```python
from build123d import *

# Parameters (mm, degrees)
F0_R     = 20
F1_DEPTH = 2
F2_R     = 5
F2_R_2   = 1.1
F3_DEPTH = 1.5


with BuildPart() as f1:
    # F0 (on Top) → F1 (new body)
    with BuildSketch(Plane.XY):
        Circle(F0_R)
        Polygon((-10.984643, -14.268413), (-5.694576, -6.98726), (-5.290067, -7.281153), (-4.885559, -7.575046), (-10.175626, -14.856199), (-10.580135, -14.562306), align=None, mode=Mode.SUBTRACT)
        Polygon((-6.037834, -16.964509), (-3.256681, -8.405), (-2.781153, -8.559509), (-2.305625, -8.714017), (-5.086778, -17.273526), (-5.562306, -17.119017), align=None, mode=Mode.SUBTRACT)
        Polygon((-14.856199, -10.175626), (-7.575046, -4.885559), (-7.281153, -5.290067), (-6.98726, -5.694576), (-14.268413, -10.984643), (-14.562306, -10.580135), align=None, mode=Mode.SUBTRACT)
        Polygon((-17.273526, -5.086778), (-8.714017, -2.305625), (-8.559509, -2.781153), (-8.405, -3.256681), (-16.964509, -6.037834), (-17.119017, -5.562306), align=None, mode=Mode.SUBTRACT)
        Polygon((-0.5, -9), (0, -9), (0.5, -9), (0.5, -18), (0, -18), (-0.5, -18), align=None, mode=Mode.SUBTRACT)
        Polygon((5.086778, -17.273526), (2.305625, -8.714017), (2.781153, -8.559509), (3.256681, -8.405), (6.037834, -16.964509), (5.562306, -17.119017), align=None, mode=Mode.SUBTRACT)
        Polygon((10.175626, -14.856199), (4.885559, -7.575046), (5.290067, -7.281153), (5.694576, -6.98726), (10.984643, -14.268413), (10.580135, -14.562306), align=None, mode=Mode.SUBTRACT)
        Polygon((14.268413, -10.984643), (6.98726, -5.694576), (7.281153, -5.290067), (7.575046, -4.885559), (14.856199, -10.175626), (14.562306, -10.580135), align=None, mode=Mode.SUBTRACT)
        Polygon((16.964509, -6.037834), (8.405, -3.256681), (8.559509, -2.781153), (8.714017, -2.305625), (17.273526, -5.086778), (17.119017, -5.562306), align=None, mode=Mode.SUBTRACT)
        Polygon((-18, 0.5), (-9, 0.5), (-9, 0), (-9, -0.5), (-18, -0.5), (-18, 0), align=None, mode=Mode.SUBTRACT)
        Polygon((-16.964509, 6.037834), (-8.405, 3.256681), (-8.559509, 2.781153), (-8.714017, 2.305625), (-17.273526, 5.086778), (-17.119017, 5.562306), align=None, mode=Mode.SUBTRACT)
        Polygon((-14.268413, 10.984643), (-6.98726, 5.694576), (-7.281153, 5.290067), (-7.575046, 4.885559), (-14.856199, 10.175626), (-14.562306, 10.580135), align=None, mode=Mode.SUBTRACT)
        Polygon((-10.175626, 14.856199), (-4.885559, 7.575046), (-5.290067, 7.281153), (-5.694576, 6.98726), (-10.984643, 14.268413), (-10.580135, 14.562306), align=None, mode=Mode.SUBTRACT)
        Polygon((-5.086778, 17.273526), (-2.305625, 8.714017), (-2.781153, 8.559509), (-3.256681, 8.405), (-6.037834, 16.964509), (-5.562306, 17.119017), align=None, mode=Mode.SUBTRACT)
        with BuildLine():
            ThreePointArc((-1.908566, -1.86), (-2.665, 0), (-1.908566, 1.86))
            Line((-1.908566, 1.86), (1.908566, 1.86))
            ThreePointArc((1.908566, 1.86), (2.665, 0), (1.908566, -1.86))
            Line((1.908566, -1.86), (-1.908566, -1.86))
        make_face(mode=Mode.SUBTRACT)
        Polygon((18, -0.5), (9, -0.5), (9, 0), (9, 0.5), (18, 0.5), (18, 0), align=None, mode=Mode.SUBTRACT)
        Polygon((17.273526, 5.086778), (8.714017, 2.305625), (8.559509, 2.781153), (8.405, 3.256681), (16.964509, 6.037834), (17.119017, 5.562306), align=None, mode=Mode.SUBTRACT)
        Polygon((14.856199, 10.175626), (7.575046, 4.885559), (7.281153, 5.290067), (6.98726, 5.694576), (14.268413, 10.984643), (14.562306, 10.580135), align=None, mode=Mode.SUBTRACT)
        Polygon((0.5, 18), (0.5, 9), (0, 9), (-0.5, 9), (-0.5, 18), (0, 18), align=None, mode=Mode.SUBTRACT)
        Polygon((6.037834, 16.964509), (3.256681, 8.405), (2.781153, 8.559509), (2.305625, 8.714017), (5.086778, 17.273526), (5.562306, 17.119017), align=None, mode=Mode.SUBTRACT)
        Polygon((10.984643, 14.268413), (5.694576, 6.98726), (5.290067, 7.281153), (4.885559, 7.575046), (10.175626, 14.856199), (10.580135, 14.562306), align=None, mode=Mode.SUBTRACT)
    extrude(amount=F1_DEPTH)

    # F2 (on Top) → F3 (join)
    with BuildSketch(Plane.XY):
        Circle(F2_R)
        Circle(F2_R_2, mode=Mode.SUBTRACT)
    extrude(amount=-F3_DEPTH)


solid = f1.part
```
Check sheet for the modelled part. Datum: model origin and axes. Units: mm. A direction names the side the tool comes from. Round coordinates to 2 decimals unless told otherwise and drop trailing zeros. Loops run counter-clockwise (first coordinate to the right, second up) from the corner with the lowest first, then second, coordinate; pieces in that order, holes last. Notation, with made-up numbers: (81, 21.25) - (112, 21.25) arc R31 cw to (112, 52.25) - close; hole circle Ø5 at (10.25, 47). An arc over 180 degrees is marked (long way). Write item = value, one per line. Start each with the question number.
Q1. Release check for a two-part mould opening along Y. For faces 1 (the face through (0.5, -13, 1)), 2 (the face through (4, -4, 0)) record: pulls with the +Y half, pulls with the -Y half, needs draft (parallel to the pull), parting line crosses it, or undercut.
Q2. Access from +Z, -Z, +X, -X, +Y, -Y to the whole of each face (thin tool, end or side, straight path). Record for faces 3 (the face through (0, -1.86, 1)), 4 (the face through (0, -9, 1)).
Q3. Thickness scan on L1, parallel to Y at x = 0, z = -0.7; L2, parallel to Z at x = -2, y = 10; L3, parallel to Y at x = 8, z = 0.5. Record the ranges inside material, lowest first.
Q4. Section check C-C (z = -0.5). Record the boundary of the cut face in (x, y), plus the area to 3 significant figures.
Q5. Section check A-A (y = 0). Record the boundary of the cut face in (x, z) (3 decimals).
Q6. Depth check by flat-ended pin: P1, Ø12, axis at x = 5, y = -8, coming from the -Z side; P2, Ø1.1, axis at x = 0, z = 1, coming from the -Y side; P3, Ø1, axis at y = 14.5, z = 1, coming from the +X side; P4, Ø3, axis at x = 14.5, y = -16, coming from the +Z side. Enter the tip coordinate at first touch or a pass-through.
Q7. Section check B-B (x = 0). Record the boundary of the cut face in (y, z).
Derived:
q1.face_1 = undercut
q1.face_2 = needs draft
q2.face_3 = +Z
q2.face_4 = +Z, -Z
q3.L1 = -5 to -1.1, 1.1 to 5
q3.L2 = 0 to 2
q3.L3 = -18.33 to -11.86, -10.16 to -6.43, -5.19 to 5.19, 6.43 to 10.16, 11.86 to 18.33
q4.outline = circle Ø10 at (0, 0); hole circle Ø2.2 at (0, 0)
q4.area = 74.7 mm^2
q5.outline = (-20, 0) - (-18, 0) - (-18, 2) - (-20, 2) - close; (-9, 0) - (-5, 0) - (-5, -1.5) - (-1.1, -1.5) - (-1.1, 0) - (-2.665, 0) - (-2.665, 2) - (-9, 2) - close; (1.1, -1.5) - (5, -1.5) - (5, 0) - (9, 0) - (9, 2) - (2.665, 2) - (2.665, 0) - (1.1, 0) - close; (18, 0) - (20, 0) - (20, 2) - (18, 2) - close
q6.P1 = -1.5
q6.P2 = -20
q6.P3 = 14.28
q6.P4 = through
q7.outline = (-20, 0) - (-18, 0) - (-18, 2) - (-20, 2) - close; (-9, 0) - (-5, 0) - (-5, -1.5) - (-1.1, -1.5) - (-1.1, 0) - (-1.86, 0) - (-1.86, 2) - (-9, 2) - close; (1.1, -1.5) - (5, -1.5) - (5, 0) - (9, 0) - (9, 2) - (1.86, 2) - (1.86, 0) - (1.1, 0) - close; (18, 0) - (20, 0) - (20, 2) - (18, 2) - close
